Can you work these out from the model? Positions are in its coordinate system, mm. A direction names the side the tool comes from. Coordinates: 2 decimals unless noted, no trailing zeros. Order: outer loops, then holes, each group sorted by start corner. A loop starts at its lowest first (then second) coordinate and runs counter-clockwise, first axis right, second up. Notation, with made-up numbers: (50, 50) -> (83, 50) arc R16 cw to (83, 80) -> close; hole circle Ø5 at (63, 7). An arc over 180 degrees is marked (long way). Write item = value, one per line.
Autodesk Inventor part; units mm, degrees
ref_plane "YZ Plane" through (0, 0, 0) normal (1, 0, 0) x (0, 1, 0)
ref_plane "XZ Plane" through (0, 0, 0) normal (0, 1, 0) x (-1, 0, 0)
ref_plane "XY Plane" through (0, 0, 0) normal (0, 0, 1) x (1, 0, 0)
sketch "Szkic1" plane through (0, 0, 0) normal (0, 1, 0) x (-1, 0, 0)
  circle A0 centre (0, 0) radius 10.875
  circle A1 centre (0, 0) radius 4
  point P0 (8, 0)
  point P1 (0, -8)
  point P2 (-8, 0)
  point P3 (0, 8)
  dimension "d0" = 21.75
  dimension "d1" = 8
  dimension "d2" = 8
  dimension "d5" = 360
extrude "Wyciągnięcie proste1" add sketch "Szkic1" along normal blind 4
sketch "Szkic2" plane through (0, 4, 0) normal (0, 1, 0) x (1, 0, 0)
  circle A0 centre (0, 0) radius 4
  circle A1 centre (0, 0) radius 10.875
  point P0 (-8, 0)
  point P1 (0, -8)
  point P2 (8, 0)
  point P3 (0, 8)
  dimension "d11" = 360
  dimension "d20" = 8
hole "Otwór1" at (-8, 4, 0) at (0, 4, 8) at (8, 4, 0) at (0, 4, -8) direction (0, -1, 0) diameter 3.2 end through all
sketch "Szkic3" plane through (0, 0, 0) normal (0, -1, 0) x (1, 0, 0)
  circle A0 centre (0, 0) radius 5.17
  circle A1 centre (0, 0) radius 4
  dimension "d21" = 10.34
extrude "Wyciągnięcie proste2" add sketch "Szkic3" along normal blind 10.8
sketch "Szkic4" plane through (0, 0, 0) normal (1, 0, 0) x (0, 1, 0)
  line L0 (-10.8, 5.17) -> (-7.3, 5.17)
  line L1 (-7.3, 5.17) -> (-7.3, -5.17)
  line L2 (-7.3, -5.17) -> (-10.8, -5.17)
  line L3 (-10.8, -5.17) -> (-10.8, 5.17)
  line L4 (0, -5.17) -> (0, 5.17)
  line L5 (-10.8, -4) -> (-10.8, 4)
  line L6 (0, 5.17) -> (-10.8, 5.17)
  line L7 (0, -5.17) -> (-10.8, -5.17)
  line L8 (-10.8, 0) -> (4, 0)
  line L9 (4, -10.875) -> (4, 10.875)
  point P0 (0, 0)
  dimension "d24" = 10.34
  dimension "d25" = 7.3
  dimension "d26" = 10.34
extrude "Wyciągnięcie proste3" cut sketch "Szkic4" along normal mid plane 3.9 contours L0 L1 L8 L3 | L1 L2 L3 L8
equation "\"d24\" = d26"
properties part number "TR8_AntiBacklashNutMain"
Item 1: I want a section at C-C, the plane y = -8. Please give me the cut outline in (x, z), plus the area to 3 significant figures.
A:
outline = (-1.95, -4.79) -> (-1.95, -3.49) arc R4 cw to (-1.95, 3.49) -> (-1.95, 4.79) arc R5.17 ccw to start; (1.95, -4.79) arc R5.17 ccw to (1.95, 4.79) -> (1.95, 3.49) arc R4 cw to (1.95, -3.49) -> close
area = 24.3 mm2
Item 2: I want a section at D-D, the plane x = -2.25. Please give me the cut outline in (y, z), plus the area to 3 significant figures.
A:
outline = (-10.8, -4.65) -> (0, -4.65) -> (0, -10.64) -> (4, -10.64) -> (4, -3.31) -> (-10.8, -3.31) -> close; (-10.8, 3.31) -> (4, 3.31) -> (4, 10.64) -> (0, 10.64) -> (0, 4.65) -> (-10.8, 4.65) -> close
area = 87.8 mm2
Item 3: I'm going to push flat-ended pins straight in: P1, Ø1.5, axis at x = -5.5, y = -6.5, coming from the -Z side; P2, Ø4, axis at x = 0, z = 8, coming from the -Y side; P3, Ø6, axis at x = -5.5, y = -1.5, coming from the -Z side. Where does each tip first touch, or does it pass through?
A:
P1 = -2.04
P2 = 0
P3 = -10.48
Item 4: If I drill on probe 1 along Z at (x, y) = (0, 3) (3 decimals); probe 2 along Y at (x, z) = (9, -1.5); probe 3 along X at (y, z) = (-5.75, 0), over which ranges is the centre line in solid material (lowest first)?
A:
probe_1 = -10.875 to -9.6, -6.4 to -4, 4 to 6.4, 9.6 to 10.875
probe_2 = 0 to 4
probe_3 = -5.17 to -4, 4 to 5.17
Item 5: For faces 5 (the flat face through (1.95, -9, -4)), 6 (the flat face through (-5, 0, -2)), 7 (the cylindrical face through (1.42, 1.97, -10.78)), which set-ups out of +Z, -Z, +X, -X, +Y, -Y let a thin tool reach every point of the face, with its end or its side?
A:
face_5 = +Z, -Z, -Y
face_6 = -Y
face_7 = +Y, -Y
Item 6: If we mould it in two halves opening along X, with no side actions, what happens to faces 1 (the flat face through (0, 4, -5)), 2 (the flat face through (-1.95, -9, 4)), 3 (the flat face through (-1.95, -9, -4)), 4 (the cylindrical face through (4.931, -5.324, -1.553))? For each: pulls with the +X half, pulls with the -X half, needs draft (parallel to the pull), parting line crosses it, or undercut.
A:
face_1 = needs draft
face_2 = undercut
face_3 = undercut
face_4 = parting line crosses it
Item 7: I want a section at A-A, the plane x = 0. Please give me the cut outline in (y, z) (3 decimals), plus the area to 3 significant figures.
A:
outline = (-7.3, -5.17) -> (0, -5.17) -> (0, -6.4) -> (4, -6.4) -> (4, -4) -> (-7.3, -4) -> close; (-7.3, 4) -> (4, 4) -> (4, 6.4) -> (0, 6.4) -> (0, 5.17) -> (-7.3, 5.17) -> close; (0, -10.875) -> (4, -10.875) -> (4, -9.6) -> (0, -9.6) -> close; (0, 9.6) -> (4, 9.6) -> (4, 10.875) -> (0, 10.875) -> close
area = 46.5 mm2
Item 8: I want a section at B-B, the plane z = -8.25. Please give me the cut outline in (x, y), plus the area to 3 significant figures.
A:
outline = (-7.09, 0) -> (-1.58, 0) -> (-1.58, 4) -> (-7.09, 4) -> close; (1.58, 0) -> (7.09, 0) -> (7.09, 4) -> (1.58, 4) -> close
area = 44.0 mm2
